The drawing under review shows one solid part. Ordinate dimensions are in mm from its lowest x, y, z. A direction names the side the tool comes from. Coordinates: 2 decimals unless noted, no trailing zeros. Write each loop counter-clockwise with the first axis right and the second up, starting at its lowest first coordinate (ties: lowest second). Pieces come first, ordered by that corner, then holes. Notation, with made-up numbers: (76, 14.25) - (108, 14.25) arc R20 ccw to (108, 31.25) - close; hole circle Ø11 at (21.25, -24). An arc over 180 degrees is marked (long way). Put each result on its own line as item: value. Start each with the question number.
Item 1: For pin 1 (4 mm diameter, centred on x = 60, z = 18, fed in from -Y); pin 2 (2 mm diameter, centred on y = 33, z = 10.5, fed in from -X); pin 3 (11 mm diameter, centred on y = 24.5, z = 19, fed in from +X), all flat-tipped, find the tip position at first contact; note any pin that passes through.
Item 2: To check wall thickness, follow L1, parallel to X at y = 19.5, z = 30; L2, parallel to X at y = 7.5, z = 21; L3, parallel to Z at x = 29.5, y = 18. State the ranges of each line that lie inside material, in increasing order. Write a range as [from, to].
Item 3: Consider section D-D on y = 31.5. Give the boundary of the cut face in (x, z), then the cut area to 3 significant figures.
Item 4: Consider section B-B on z = 10. Give the boundary of the cut face in (x, y), then the cut area to 3 significant figures.
Item 5: Machinability: for the marked faces 1, 2 and 3, which of the approach directions +Z, -Z, +X, -X, +Y, -Y give a long, thin tool a straight path to every point of the face, cutting with its end or side? Answer none if there is none.
Item 6: Consider section C-C on x = 44.5. Give the boundary of the cut face in (y, z), then the cut area to 3 significant figures.
Item 7: Consider section A-A on y = 18.5. Give the boundary of the cut face in (x, z).
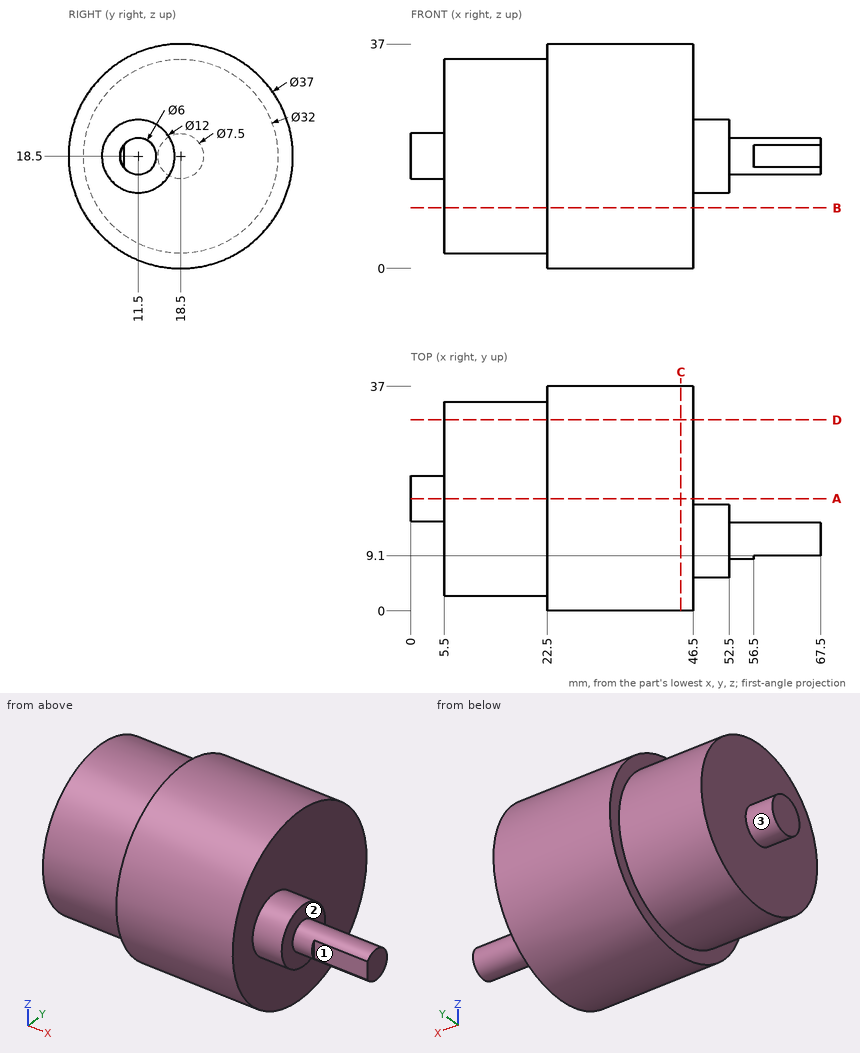
Report:
1. pin 1: y = 9.1
1. pin 2: x = 5.5
1. pin 3: x = 46.5
2. L1: [5.5, 46.5]
2. L2: [5.5, 52.5]
2. L3: [0.01, 36.99]
3. outline: (5.5, 9.17) - (22.5, 9.17) - (22.5, 5.34) - (46.5, 5.34) - (46.5, 31.66) - (22.5, 31.66) - (22.5, 27.83) - (5.5, 27.83) - close
3. area: 949 mm²
4. outline: (5.5, 4.94) - (22.5, 4.94) - (22.5, 2.07) - (46.5, 2.07) - (46.5, 34.93) - (22.5, 34.93) - (22.5, 32.06) - (5.5, 32.06) - close
4. area: 1,250 mm²
5. face 1: +Z, -Z, +X, -Y
5. face 2: +X
5. face 3: -X
6. outline: circle Ø37 at (18.5, 18.5)
6. area: 1,080 mm²
7. outline: (0, 14.75) - (5.5, 14.75) - (5.5, 2.5) - (22.5, 2.5) - (22.5, 0) - (46.5, 0) - (46.5, 37) - (22.5, 37) - (22.5, 34.5) - (5.5, 34.5) - (5.5, 22.25) - (0, 22.25) - close
